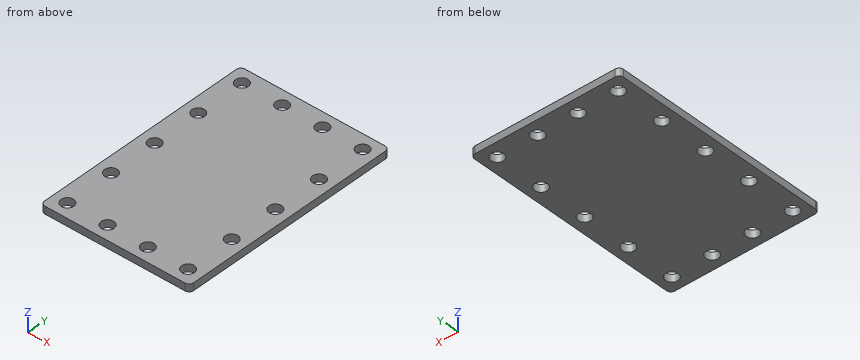
Autodesk Inventor part; units mm, degrees
ref_plane "YZ Plane" through (0, 0, 0) normal (1, 0, 0) x (0, 1, 0)
ref_plane "XZ Plane" through (0, 0, 0) normal (0, 1, 0) x (-1, 0, 0)
ref_plane "XY Plane" through (0, 0, 0) normal (0, 0, 1) x (1, 0, 0)
sketch "Sketch2" plane through (0, 0, 0) normal (0, 0, 1) x (1, 0, 0)
  line L0 (-50, -100) -> (50, -100)
  line L1 (50, -100) -> (50, 100)
  line L2 (50, 100) -> (-50, 100)
  line L3 (-50, 100) -> (-50, -100)
  line L4 (-50, -100) -> (50, 100) construction
  line L5 (50, -100) -> (-50, 100) construction
  line L6 (-100, -150) -> (100, -150)
  line L7 (100, -150) -> (100, 150)
  line L8 (100, 150) -> (-100, 150)
  line L9 (-100, 150) -> (-100, -150)
  point P0 (0, 0)
  dimension "d29" = 100
  dimension "d30" = 200
  dimension "d31" = 50
extrude "Plate2" add sketch "Sketch2" along normal blind 10 contours L3 L2 L1 L0 | L9 L8 L7 L6
sketch "Sketch5" plane through (0, 0, 10) normal (0, 0, 1) x (1, 0, 0)
  line L0 (100, -150) -> (-100, -150) construction
  line L1 (100, 150) -> (100, -150) construction
  line L2 (-100, 150) -> (100, 150) construction
  line L3 (-100, -150) -> (-100, 150) construction
  line L4 (-81, 131) -> (81, 131) construction
  line L5 (81, 131) -> (81, -131) construction
  line L6 (81, -131) -> (-81, -131) construction
  line L7 (-81, -131) -> (-81, 131) construction
  circle A0 centre (-81, -131) radius 8.5
  circle A1 centre (-81, 131) radius 8.5
  circle A2 centre (-81, 0) radius 8.5
  circle A3 centre (-81, -65.5) radius 8.5
  circle A4 centre (-81, 65.5) radius 8.5
  line L8 (-50, 0) -> (50, 0) construction
  circle A5 centre (-27, -131) radius 8.5
  circle A6 centre (-27, -65.5) radius 8.5
  circle A7 centre (-27, 0) radius 8.5
  circle A8 centre (-27, 65.5) radius 8.5
  circle A9 centre (-27, 131) radius 8.5
  circle A10 centre (27, -131) radius 8.5
  circle A11 centre (27, -65.5) radius 8.5
  circle A12 centre (27, 0) radius 8.5
  circle A13 centre (27, 65.5) radius 8.5
  circle A14 centre (27, 131) radius 8.5
  circle A15 centre (81, -131) radius 8.5
  circle A16 centre (81, -65.5) radius 8.5
  circle A17 centre (81, 0) radius 8.5
  circle A18 centre (81, 65.5) radius 8.5
  circle A19 centre (81, 131) radius 8.5
  point P0 (0, 0)
  point P1 (0, -131)
  dimension "d33" = 17
  dimension "d34" = 19
  dimension "d35" = 65.5
  dimension "d36" = 65.5
  dimension "d39" = 54
extrude "Cut3" cut sketch "Sketch5" against normal blind 10 contours A0 | A1 | A2 | A3 | A4 | A5 | A9 | A10 | A14 | A15 | A16 | A17 | A18 | A19
fillet "Corner Round1" radius 6 4 edges at (-100, -150, 5) (-100, 150, 5) (100, 150, 5) (100, -150, 5)
equation "\"d35\" = d36"
equation "\"d44\" = Thickness"
equation "\"d14\" = Thickness"
equation "\"BendReliefDepth\" = 0.5 * Thickness"
equation "\"TransitionRadius\" = BendRadius"
equation "\"JacobiRadiusSize\" = BendRadius"
properties part number "PNS 1607 charging flange rect_1200" material "Steel"
CAD build for the part. Positions are in the model's coordinates, mm. Give positions to 0.01 mm unless a question says otherwise; leave off trailing zeros. Loops run counter-clockwise (first coordinate to the right, second up) from the corner with the lowest first, then second, coordinate; pieces in that order, holes last. Notation, with made-up numbers: M 53.5,-36.5 L 104.5,-36.5 A21 cw 104.5,-3.5 Z; hole C -17,13 d10. An arc over 180 degrees is marked long. One line per question, with ' | ' between items. Start each with the question number.
1. Probe L1, parallel to Y at x = 81, z = 7.75; L2, parallel to Y at x = 27, z = 4; L3, parallel to Y at x = -26, z = 8.75. List the from-to ranges inside material, lowest first. Write a range as from..to.
2. Saw through at D-D on x = -32. Give the cut face in (y, z), plus the area to 3 significant figures.
3. Saw through at A-A on y = -131. Give the cut face in (x, z), plus the area to 3 significant figures.
4. Saw through at B-B on z = 6.5. State how many separate pieces and enclosed holes the cut face has, plus the area to 3 significant figures.
5. Saw through at C-C on y = -65.5. Give the cut face in (x, z).
Result sheet:
1) L1: y = -150..-139.5, -122.5..-74, -57..-8.5, 8.5..57, 74..122.5, 139.5..150 | L2: y = -150..-139.5, -122.5..122.5, 139.5..150 | L3: y = -150..-139.44, -122.56..122.56, 139.44..150
2) outline: M -150,0 L -137.87,0 L -137.87,10 L -150,10 Z; M -124.13,0 L 124.13,0 L 124.13,10 L -124.13,10 Z; M 137.87,0 L 150,0 L 150,10 L 137.87,10 Z | area: 2,730 mm^2
3) outline: M -100,0 L -89.5,0 L -89.5,10 L -100,10 Z; M -72.5,0 L -35.5,0 L -35.5,10 L -72.5,10 Z; M -18.5,0 L 18.5,0 L 18.5,10 L -18.5,10 Z; M 35.5,0 L 72.5,0 L 72.5,10 L 35.5,10 Z; M 89.5,0 L 100,0 L 100,10 L 89.5,10 Z | area: 1,320 mm^2
4) separate pieces: 1 | enclosed holes: 14 | area: 56,800 mm^2
5) outline: M -100,0 L -89.5,0 L -89.5,10 L -100,10 Z; M -72.5,0 L 72.5,0 L 72.5,10 L -72.5,10 Z; M 89.5,0 L 100,0 L 100,10 L 89.5,10 Z
